CAD build for the part. Positions are in the model's coordinates, mm. Face numbers are marked on the shaded views. A direction names the side the tool comes from. Coordinates: 2 decimals unless noted, no trailing zeros. Order: outer loops, then holes, each group sorted by start corner. A loop starts at its lowest first (then second) coordinate and runs counter-clockwise, first axis right, second up. Notation, with made-up numbers: M 10,88 L 47,88 A22 ccw 47,125 Z; hole C 62,-32.5 d1. An arc over 180 degrees is marked long. Write item = value, one per line.
from build123d import *

# Parameters (mm, degrees)
EXTRUDED_BOSS_FRONT_PLANE_WING_DEPTH      = 8.89
EXTRUDED_BOSS_FRONT_PLANE_WING_DEPTH_BACK = 8.89
EXTRUDED_CUT_RIGHT_PLANE_WING_DEPTH       = 31.926520981
EXTRUDED_CUT_RIGHT_PLANE_WING_DEPTH_BACK  = 31.926520981
SKETCH3_W                                 = 16.002
SKETCH3_H                                 = 14.351
F_2X_0_2D_HOLES_D                         = 5.08
F_0_35D_HOLE_D                            = 8.89
F_0_135D_HOLE_D                           = 3.429
F_0_135D_HOLE_DEPTH                       = 0.889
F_0_2D_0_135D_HOLE_CONNECTING_CUT_DEPTH   = 35.098731369
INNER_CONNECTING_FILLET_R                 = 0.254
OUTTER_CONNECTING_FILLET_R                = 1.016


with BuildPart() as part:
    # Sketch2 → Extruded Boss Front Plane Wing (new, two sides: drawn at the far end of the back side and taken through both)
    with BuildSketch(Plane.XY.offset(-EXTRUDED_BOSS_FRONT_PLANE_WING_DEPTH_BACK)):
        with BuildLine():
            Line((-19.05, 0), (19.05, 0))
            Line((19.05, 0), (19.05, 5.08))
            Line((19.05, 5.08), (-19.05, 15.24))
            ThreePointArc((-19.05, 15.24), (-25.4, 8.89), (-19.05, 2.54))
            Line((-19.05, 2.54), (-19.05, 0))
        make_face()
    extrude(amount=EXTRUDED_BOSS_FRONT_PLANE_WING_DEPTH + EXTRUDED_BOSS_FRONT_PLANE_WING_DEPTH_BACK)

    # Sketch3 → Extruded Cut Right Plane Wing (cut, two sides: drawn at the far end of the back side and taken through both)
    with BuildSketch(Plane(origin=(0, 0, 0), x_dir=(0, 0, -1), z_dir=(1, 0, 0)).offset(-EXTRUDED_CUT_RIGHT_PLANE_WING_DEPTH_BACK)):
        with Locations((0, 8.0645)):
            Rectangle(SKETCH3_W, SKETCH3_H)
    extrude(amount=EXTRUDED_CUT_RIGHT_PLANE_WING_DEPTH + EXTRUDED_CUT_RIGHT_PLANE_WING_DEPTH_BACK, mode=Mode.SUBTRACT)

    # 2X 0.2D Holes (through all)
    with Locations(Plane.XY.offset(8.89)):
        with Locations((-19.05, 8.89)):
            Hole(F_2X_0_2D_HOLES_D / 2)

    # 0.35D Hole (through all)
    with Locations(Plane(origin=(0, 0.889, 0), x_dir=(1, 0, 0), z_dir=(0, 1, 0))):
        with Locations((-19.05, 0)):
            Hole(F_0_35D_HOLE_D / 2)

    # 0.135D Hole
    with Locations(Plane.XY.offset(-8.001)):
        with Locations((-5.7785, 5.08)):
            Hole(F_0_135D_HOLE_D / 2, depth=F_0_135D_HOLE_DEPTH)

    # Sketch14 → 0.2D-0.135D Hole Connecting Cut (cut, through all)
    with BuildSketch(Plane.XY.offset(-8.001)):
        Polygon((-19.603662053, 6.411077183), (-6.152221886, 3.406727099), (-5.207730823, 6.696704301), (-18.204416034, 11.285117483), align=None)
    extrude(amount=-F_0_2D_0_135D_HOLE_CONNECTING_CUT_DEPTH, mode=Mode.SUBTRACT)

    # Inner Connecting Fillet
    inner_connecting_fillet_edges = [part.edges().sort_by_distance(p)[0] for p in [
        (19.05, 5.08, 8.4455),
        (0, 0.889, -8.001),
        (0, 0.889, 8.001),
        (19.05, 5.08, -8.4455),
    ]]
    fillet(inner_connecting_fillet_edges, radius=INNER_CONNECTING_FILLET_R)

    # Outter Connecting Fillet
    outter_connecting_fillet_edges = [part.edges().sort_by_distance(p)[0] for p in [
        (0, 0, 8.89),
        (0, 0, -8.89),
    ]]
    fillet(outter_connecting_fillet_edges, radius=OUTTER_CONNECTING_FILLET_R)


solid = part.part
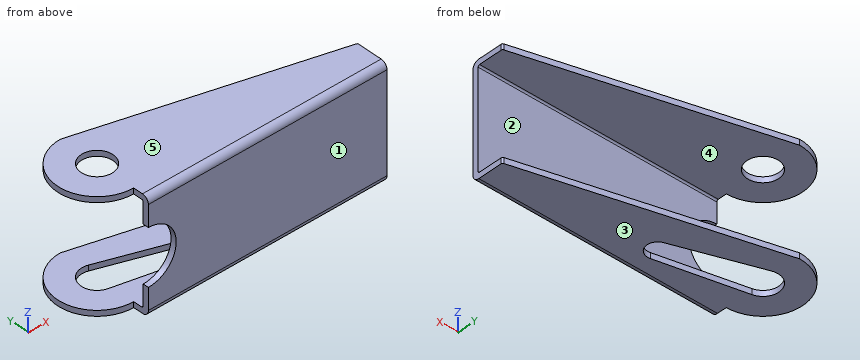
(1) Pull direction Z, two halves, no side cores. Call the marked faces 1, 2 and 3: +Z half, -Z half, draft (parallel to the pull), parting line (faces both ways), or undercut.
Evaluation:
face_1 = draft
face_2 = undercut
face_3 = -Z half
(2) Wall check: line 1 (Z direction, x = 1.5, y = 7.5); line 2 (Z direction, x = -16.5, y = 7); line 3 (Y direction, x = 12.5, z = 6.75). Give the ranges that are in metal, low to high. Write a range as from..to.
Evaluation:
line_1 = -8.89..-8, 8..8.89
line_2 = 8..8.89
line_3 = 0..0.89
(3) Pin check, flat tips, straight feed: pin 1 Ø3 at (y, z) = (0.5, 6.5) entering from -X; pin 2 Ø2 at (x, z) = (12, 4) entering from +Y. Stop position of each tip, or through.
Evaluation:
pin_1 = -19.05
pin_2 = 0.89
(4) Slice it at D-D, the plane z = 6.5. Write the cut outline in (x, y).
Evaluation:
outline = M -19.05,0 L 19.05,0 L 19.05,0.89 L -19.05,0.89 Z
(5) Slice it at C-C, the plane x = -20.5. Write the cut outline in (y, z), then the cut area to 3 significant figures.
Evaluation:
outline = M 2.71,-8.89 L 6.8,-8.89 L 6.8,-8 L 2.71,-8 Z; M 2.71,8 L 6.8,8 L 6.8,8.89 L 2.71,8.89 Z; M 10.98,-8.89 L 15.07,-8.89 L 15.07,-8 L 10.98,-8 Z; M 10.98,8 L 15.07,8 L 15.07,8.89 L 10.98,8.89 Z
area = 14.6 mm²
(6) Slice it at A-A, the plane y = 1.75. Write the cut outline in (x, z).
Evaluation:
outline = M -19.05,-8.89 L 19.05,-8.89 L 19.05,-8 L -19.05,-8 Z; M -19.05,8 L 19.05,8 L 19.05,8.89 L -19.05,8.89 Z
(7) Slice it at B-B, the plane y = 7.75. Write the cut outline in (x, z).
Evaluation:
outline = M -25.3,-8.89 L -21.32,-8.89 L -21.32,-8 L -25.3,-8 Z; M -25.3,8 L -21.32,8 L -21.32,8.89 L -25.3,8.89 Z; M -16.78,8 L 9.04,8 L 9.04,8.89 L -16.78,8.89 Z; M -8.19,-8.89 L 9.04,-8.89 L 9.04,-8 L -8.19,-8 Z
(8) Tool access for the marked faces 4 and 5: list every direction of +Z, -Z, +X, -X, +Y, -Y with a clear straight run to the whole face (end or side of a thin tool).
Evaluation:
face_4 = +X, -X, +Y
face_5 = +Z, +X, -X, +Y, -Y
